Source: CAD feature listing. Evaluate the final solid. Frame: model axes, mm. A direction names the side the tool comes from. Round coordinates to 2 decimals unless told otherwise and drop trailing zeros. Loops run counter-clockwise (first coordinate to the right, second up) from the corner with the lowest first, then second, coordinate; pieces in that order, holes last. Notation, with made-up numbers: (57, 78) - (106, 78) arc R13 cw to (106, 88) - close; hole circle Ø6 at (21, 25). An arc over 180 degrees is marked (long way). Write item = value, one per line. Start each with the question number.
from build123d import *

# Parameters (mm, degrees)
F0_W     = 145
F0_H     = 580
F1_DEPTH = 3
F2_W     = 145
F2_H     = 580
F2_W_2   = 138.9999985695
F2_H_2   = 573.9999985695
F3_DEPTH = 30
F4_W     = 125
F4_H     = 560
F4_W_2   = 119.0000200272
F4_H_2   = 554.0000200272
F5_DEPTH = 10
F6_R     = 0.5


with BuildPart() as f1:
    # F0 (on Top) → F1 (new body)
    with BuildSketch(Plane.XY):
        Rectangle(F0_W, F0_H)
    extrude(amount=F1_DEPTH)

    # F2 (on face) → F3 (join)
    with BuildSketch(Plane.XY.offset(3)):
        Rectangle(F2_W, F2_H)
        Rectangle(F2_W_2, F2_H_2, mode=Mode.SUBTRACT)
    extrude(amount=F3_DEPTH)

    # F4 (on face) → F5 (join)
    with BuildSketch(Plane(origin=(0, 0, 0), x_dir=(1, 0, 0), z_dir=(0, 0, -1))):
        Rectangle(F4_W, F4_H)
        Rectangle(F4_W_2, F4_H_2, mode=Mode.SUBTRACT)
    extrude(amount=F5_DEPTH)

    # F6
    f6_edges = [f1.edges().sort_by_distance(p)[0] for p in [
        (0, 290, 0),
        (72.5, 0, 0),
        (-72.5, 0, 0),
        (0, -290, 0),
        (62.5, 0, 0),
        (0, 280, 0),
        (-62.5, 0, 0),
        (0, -280, 0),
        (59.50001, 0, 0),
        (0, -277.00001, 0),
        (-59.50001, 0, 0),
        (0, 277.00001, 0),
        (-62.5, 280, -5),
        (0, -280, -10),
        (-62.5, 0, -10),
        (0, 280, -10),
        (62.5, 0, -10),
        (0, 277.00001, -10),
        (-59.50001, 0, -10),
        (0, -277.00001, -10),
        (59.50001, 0, -10),
        (59.50001, 277.00001, -5),
        (-59.50001, 277.00001, -5),
        (62.5, -280, -5),
        (-62.5, -280, -5),
        (62.5, 280, -5),
        (-72.5, -290, 16.5),
        (0, -290, 33),
        (72.5, -290, 16.5),
        (72.5, 0, 33),
        (72.5, 290, 16.5),
        (0, 290, 33),
        (-72.5, 290, 16.5),
        (69.499999, 0, 33),
        (0, 286.999999, 3),
        (-69.499999, -286.999999, 18),
        (-69.499999, 286.999999, 18),
        (-69.499999, 0, 3),
        (-69.499999, 0, 33),
        (69.499999, -286.999999, 18),
        (0, -286.999999, 3),
        (0, -286.999999, 33),
        (-72.5, 0, 33),
        (0, 286.999999, 33),
    ]]
    fillet(f6_edges, radius=F6_R)


solid = f1.part
(1) Cut plane A-A (z = 22.5). Output: boundary loops of the cut face in (x, y), and give its area (3 significant figures).
(2) Access query for faces 5 (the face through (-62.5, 4, -5)), 6 (the face through (-1, -277, -5)), 7 (the face through (-1, 4, 3)). Directions: +Z, -Z, +X, -X, +Y, -Y. A direction counts if a zero-diameter tool reaches every point of the face in a straight line with its end or side. Return the directions, or none.
(3) Material intervals for line 1 along X through (y, z) = (42.5, -4); line 2 along Y through (x, z) = (-8, 25.5); line 3 along X through (y, z) = (-54, 15.5), sorted ascending. Write a range as from..to.
(4) Mould query, pull axis Y, two halves, no side actions, for faces 1 (the face through (-1, -287, 18)), 2 (the face through (62.5, 4, -5)), 3 (the face through (-69.5, -4, 18)), 4 (the face through (-1, 290, 16)). Classes: +Y half, -Y half, draft (parallel to the pull), parting line (faces both ways), or undercut.
(5) Pin query (flat end, axial travel): P1, Ø10, axis at x = 0.5, z = -3.5, coming from the +Y side; P2, Ø6, axis at x = -12, y = -50, coming from the -Z side; P3, Ø2.5, axis at x = 30, z = -4, coming from the +Y side; P4, Ø4.5, axis at x = 17.5, z = -6, coming from the -Y side. Return the tip coordinate at first contact, or that it passes through.
Solution:
q1.outline = (-72.5, -289.5) arc R0.5 ccw to (-72, -290) - (72, -290) arc R0.5 ccw to (72.5, -289.5) - (72.5, 289.5) arc R0.5 ccw to (72, 290) - (-72, 290) arc R0.5 ccw to (-72.5, 289.5) - close; hole (-69.5, -286.5) arc R0.5 ccw to (-69, -287) - (69, -287) arc R0.5 ccw to (69.5, -286.5) - (69.5, 287) - (-69, 287) arc R0.5 ccw to (-69.5, 286.5) - close
q1.area = 4,310 mm^2
q2.face_5 = -Z, -X, +Y, -Y
q2.face_6 = -Z
q2.face_7 = +Z
q3.line_1 = -62.5..-59.5, 59.5..62.5
q3.line_2 = -290..-287, 287..290
q3.line_3 = -72.5..-69.5, 69.5..72.5
q4.face_1 = undercut
q4.face_2 = draft
q4.face_3 = undercut
q4.face_4 = +Y half
q5.P1 = 290
q5.P2 = 0
q5.P3 = 280
q5.P4 = -280
